Autodesk Inventor part; units mm, degrees
ref_plane "YZ Plane" through (0, 0, 0) normal (1, 0, 0) x (0, 1, 0)
ref_plane "XZ Plane" through (0, 0, 0) normal (0, 1, 0) x (-1, 0, 0)
ref_plane "XY Plane" through (0, 0, 0) normal (0, 0, 1) x (1, 0, 0)
sketch "Skizze1" plane through (0, 0, 0) normal (0, 0, 1) x (1, 0, 0)
  circle A0 centre (0, 0) radius 3.7 construction
  line L0 (0, 3.7) -> (3.5189, 1.1434)
  line L1 (3.5189, 1.1434) -> (2.1748, -2.9934)
  line L2 (2.1748, -2.9934) -> (-2.1748, -2.9934)
  line L3 (-2.1748, -2.9934) -> (-3.5189, 1.1434)
  line L4 (-3.5189, 1.1434) -> (0, 3.7)
  circle A1 centre (0, 0) radius 5.2 construction
  line L5 (0, 5.2) -> (4.9455, 1.6069)
  line L6 (4.9455, 1.6069) -> (3.0565, -4.2069)
  line L7 (3.0565, -4.2069) -> (-3.0565, -4.2069)
  line L8 (-3.0565, -4.2069) -> (-4.9455, 1.6069)
  line L9 (-4.9455, 1.6069) -> (0, 5.2)
  circle A2 centre (0, 0) radius 1.75
  circle A3 centre (0, 0) radius 6.5 construction
  line L10 (-6.1819, 2.0086) -> (0, 6.5)
  line L11 (0, 6.5) -> (6.1819, 2.0086)
  line L12 (6.1819, 2.0086) -> (3.8206, -5.2586)
  line L13 (3.8206, -5.2586) -> (-3.8206, -5.2586)
  line L14 (-3.8206, -5.2586) -> (-6.1819, 2.0086)
  circle A4 centre (0, 0) radius 4.2 construction
  line L15 (0, 9.1) -> (0, -9.1) construction
  circle A5 centre (0, 0) radius 5.7 construction
  dimension "d9" = 13
  dimension "d8" = 3.5
  dimension "d14" = 8.4
  dimension "d15" = 0.5
  dimension "d16" = 11.4
  dimension "d18" = 0.5
extrude "Extrusion1" add sketch "Skizze1" along normal blind 4.4 contours L5 L6 L7 L8 L9
extrude "Extrusion2" add sketch "Skizze1" along normal blind 1.5 from surface at 4.4 contours L0 L1 L2 L3 L4 | L5 L6 L7 L8 L9
extrude "Extrusion3" add sketch "Skizze1" along normal blind 2 from surface at 5.9 contours L0 L1 L2 L3 L4 | L5 L6 L7 L8 L9 | L10 L11 L12 L13 L14
properties part number "gearNotch"
The model under review builds one solid part; all positions refer to its coordinate system, in mm. A direction names the side the tool comes from. Round coordinates to 2 decimals unless told otherwise and drop trailing zeros. Loops run counter-clockwise (first coordinate to the right, second up) from the corner with the lowest first, then second, coordinate; pieces in that order, holes last. Notation, with made-up numbers: (75, -22) -> (100, -22) arc R33 ccw to (100, 15) -> close; hole circle Ø4 at (22.5, 87). An arc over 180 degrees is marked (long way). Answer in a Markdown table with one row per item.
1) For pin 1 Ø3 at (x, y) = (0, 0) entering from +Z; pin 2 Ø2 at (x, z) = (0.5, 2.5) entering from +Y; pin 3 Ø3 at (y, z) = (-2.5, 2.5) entering from +X; pin 4 Ø1.5 at (x, z) = (1.5, 4.5) entering from -Y, all flat-tipped, find the tip position at first contact; note any pin that passes through.
Taken from the geometry:
| item | result |
|---|---|
| pin 1 | passes through |
| pin 2 | stops at y = 5.2 |
| pin 3 | stops at x = 4.1 |
| pin 4 | stops at y = -4.21 |
2) Wall thickness on line 1 along X through (y, z) = (-2.25, 4.25); line 2 along X through (y, z) = (2.25, 1.25); line 3 along Y through (x, z) = (0.5, 4): over which ranges is each line inside the solid? List them lowest first.
Taken from the geometry:
| item | result |
|---|---|
| line 1 | x = -3.69 to -2.42, 2.42 to 3.69 |
| line 2 | x = -4.06 to -2, 2 to 4.06 |
| line 3 | y = -4.21 to -2.99, 3.34 to 4.84 |
3) Consider section B-B, the plane y = -0.5. Write out the cut boundary in (x, z).
Taken from the geometry:
| item | result |
|---|---|
| outline | (-5.37, 5.9) -> (-4.26, 5.9) -> (-4.26, 0) -> (-2.98, 0) -> (-2.98, 4.4) -> (-1.68, 4.4) -> (-1.68, 7.9) -> (-5.37, 7.9) -> close; (1.68, 4.4) -> (2.98, 4.4) -> (2.98, 0) -> (4.26, 0) -> (4.26, 5.9) -> (5.37, 5.9) -> (5.37, 7.9) -> (1.68, 7.9) -> close |
4) Consider section A-A, the plane x = 0.5. Write out the cut boundary in (y, z).
Taken from the geometry:
| item | result |
|---|---|
| outline | (-5.26, 5.9) -> (-4.21, 5.9) -> (-4.21, 0) -> (-2.99, 0) -> (-2.99, 4.4) -> (-1.68, 4.4) -> (-1.68, 7.9) -> (-5.26, 7.9) -> close; (1.68, 4.4) -> (3.34, 4.4) -> (3.34, 0) -> (4.84, 0) -> (4.84, 5.9) -> (6.14, 5.9) -> (6.14, 7.9) -> (1.68, 7.9) -> close |
5) Consider section C-C, the plane z = 1.75. Write out the cut boundary in (x, y), plus the area to 3 significant figures.
Taken from the geometry:
| item | result |
|---|---|
| outline | (-4.95, 1.61) -> (-3.06, -4.21) -> (3.06, -4.21) -> (4.95, 1.61) -> (0, 5.2) -> close; hole (-3.52, 1.14) -> (-2.17, -2.99) -> (2.17, -2.99) -> (3.52, 1.14) -> (0, 3.7) -> close |
| area | 31.7 mm² |
6) Draft analysis for pull direction X (two halves, no side actions). For faces 1 (the flat face through (-4, -1.3, 2.9)), 2 (the flat face through (2.856, -0.896, 2.169)), 3 (the flat face through (4, -1.3, 2.9)), state which applies: pulls with the +X half, pulls with the -X half, needs draft (parallel to the pull), parting line crosses it, or undercut.
Taken from the geometry:
| item | result |
|---|---|
| face 1 | pulls with the -X half |
| face 2 | undercut |
| face 3 | pulls with the +X half |
7) Tool access review of faces 4 (the flat face through (0, -4.207, 3)), 5 (the flat face through (0, -2.993, 2)), 6 (the flat face through (-2.507, 3.378, 2.909)): name each direction out of +Z, -Z, +X, -X, +Y, -Y from which nothing blocks a thin tool from reaching the whole face with its end or side.
Taken from the geometry:
| item | result |
|---|---|
| face 4 | -Z, +X, -X, -Y |
| face 5 | -Z |
| face 6 | -Z, -X, +Y |
8) Consider section D-D, the plane x = 2.5. Write out the cut boundary in (y, z), plus the area to 3 significant figures.
Taken from the geometry:
| item | result |
|---|---|
| outline | (-5.26, 5.9) -> (-4.21, 5.9) -> (-4.21, 0) -> (-1.99, 0) -> (-1.99, 4.4) -> (1.88, 4.4) -> (1.88, 0) -> (3.38, 0) -> (3.38, 5.9) -> (4.68, 5.9) -> (4.68, 7.9) -> (-5.26, 7.9) -> close |
| area | 47.6 mm² |
